Model file for the job. Use its own axes, mm. Coordinates: 2 decimals unless noted, no trailing zeros. Loops run counter-clockwise (first coordinate to the right, second up) from the corner with the lowest first, then second, coordinate; pieces in that order, holes last.
from build123d import *

# Parameters (mm, degrees)
SKETCH1_R           = 2.5
BOSS_EXTRUDE1_DEPTH = 9


with BuildPart() as part:
    # Sketch1 → Boss-Extrude1 (new body)
    # profile 1 of 2: a face of its own
    with BuildSketch(Plane(origin=(0, 0, 0), x_dir=(1, 0, 0), z_dir=(0, 1, 0))):
        Polygon((42.5, 102.604076401), (-42.5, 102.604076401), (-102.604076401, 42.5), (-102.604076401, -42.5), (-42.5, -102.604076401), (42.5, -102.604076401), (102.604076401, -42.5), (102.604076401, 42.5), align=None)
        with Locations(Location((-39.448264129, -95.209016687, 0), (0, 0, 270))):
            Circle(SKETCH1_R, mode=Mode.SUBTRACT)
        with BuildLine():
            Line((-59.824116139, -64.773863607), (-64.066756826, -69.016504294))
            ThreePointArc((-64.066756826, -69.016504294), (-69.016504294, -69.016504294), (-69.016504294, -64.066756826))
            Line((-69.016504294, -64.066756826), (-64.773863607, -59.824116139))
            ThreePointArc((-64.773863607, -59.824116139), (-60.95959786, -59.065411509), (-58.798989873, -62.298989873))
            ThreePointArc((-58.798989873, -62.298989873), (-59.065411509, -63.638381887), (-59.824116139, -64.773863607))
        make_face(mode=Mode.SUBTRACT)
        with Locations(Location((39.428806258, -95.217076401, 0), (0, 0, 270))):
            Circle(SKETCH1_R, mode=Mode.SUBTRACT)
        with Locations(Location((-95.217076401, -39.428806258, 0), (0, 0, 270))):
            Circle(SKETCH1_R, mode=Mode.SUBTRACT)
        with BuildLine():
            Line((64.773863607, -59.824116139), (69.016504294, -64.066756826))
            ThreePointArc((69.016504294, -64.066756826), (69.775208924, -65.202238547), (70.04163056, -66.54163056))
            ThreePointArc((70.04163056, -66.54163056), (67.881022574, -69.775208924), (64.066756826, -69.016504294))
            Line((64.066756826, -69.016504294), (59.824116139, -64.773863607))
            ThreePointArc((59.824116139, -64.773863607), (59.824116139, -59.824116139), (64.773863607, -59.824116139))
        make_face(mode=Mode.SUBTRACT)
        with Locations(Location((95.209016687, -39.448264129, 0), (0, 0, 270))):
            Circle(SKETCH1_R, mode=Mode.SUBTRACT)
        with Locations(Location((-95.209016687, 39.448264129, 0), (0, 0, 270))):
            Circle(SKETCH1_R, mode=Mode.SUBTRACT)
        with BuildLine():
            Line((-64.773863607, 59.824116139), (-69.016504294, 64.066756826))
            ThreePointArc((-69.016504294, 64.066756826), (-69.016504294, 69.016504294), (-64.066756826, 69.016504294))
            Line((-64.066756826, 69.016504294), (-59.824116139, 64.773863607))
            ThreePointArc((-59.824116139, 64.773863607), (-59.065411509, 63.638381887), (-58.798989873, 62.298989873))
            ThreePointArc((-58.798989873, 62.298989873), (-60.95959786, 59.065411509), (-64.773863607, 59.824116139))
        make_face(mode=Mode.SUBTRACT)
        with Locations(Location((-39.428806258, 95.217076401, 0), (0, 0, 270))):
            Circle(SKETCH1_R, mode=Mode.SUBTRACT)
        with Locations(Location((39.448264129, 95.209016687, 0), (0, 0, 270))):
            Circle(SKETCH1_R, mode=Mode.SUBTRACT)
        with Locations(Location((95.217076401, 39.428806258, 0), (0, 0, 270))):
            Circle(SKETCH1_R, mode=Mode.SUBTRACT)
        with BuildLine():
            Line((59.824116139, 64.773863607), (64.066756826, 69.016504294))
            ThreePointArc((64.066756826, 69.016504294), (67.881022574, 69.775208924), (70.04163056, 66.54163056))
            ThreePointArc((70.04163056, 66.54163056), (69.775208924, 65.202238547), (69.016504294, 64.066756826))
            Line((69.016504294, 64.066756826), (64.773863607, 59.824116139))
            ThreePointArc((64.773863607, 59.824116139), (59.824116139, 59.824116139), (59.824116139, 64.773863607))
        make_face(mode=Mode.SUBTRACT)
    # profile 2 of 2: a face of its own
    with BuildSketch(Plane(origin=(0, 0, 0), x_dir=(1, 0, 0), z_dir=(0, 1, 0))):
        Polygon((102.604076401, -42.5), (185.604076401, -42.5), (210.604076401, -17.5), (210.604076401, 17.5), (185.604076401, 42.5), (102.604076401, 42.5), align=None)
    extrude(amount=BOSS_EXTRUDE1_DEPTH)


solid = part.part
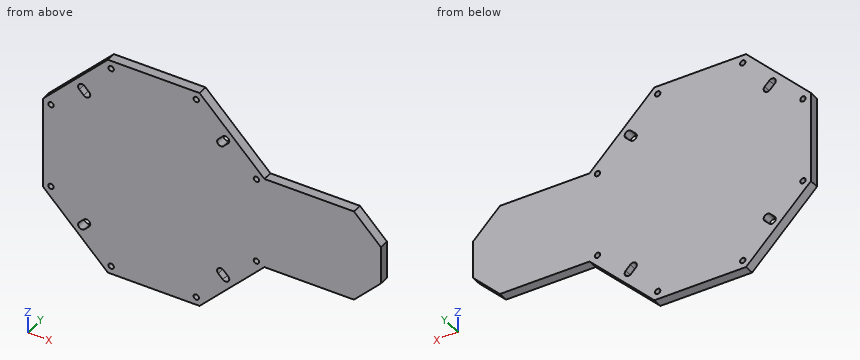
Q1. Slice it at B-B (y = 3.25). Count the separate pieces of the cut face and the enclosed holes in it, and give its area (3 significant figures).
Answers:
separate pieces: 1
enclosed holes: 12
area: 43,000 mm2
Q2. Flat gauge pins, fed straight in: P1, Ø5, axis at y = 6.5, z = 63, coming from the +X side; P2, Ø1, axis at y = 3, z = -68, coming from the +X side; P3, Ø6, axis at x = 39.43, z = 95.22, coming from the +Y side; P4, Ø4, axis at y = 6.5, z = -54, coming from the +X side. Where does each tip first touch, or does it go through?
Answers:
P1: stops at x = 84.6
P2: stops at x = 77.6
P3: stops at y = 9
P4: stops at x = 93.1
Q3. Drill centre lines: line 1 (X direction, y = 8.5, z = -68); line 2 (Z direction, x = 67, y = 5); line 3 (Z direction, x = 63, y = 6). Where is each one in solid material? Low to high.
Answers:
line 1: x = -77.1 to -69.72, -63.05 to 63.05, 69.72 to 77.1
line 2: z = -78.1 to -70.01, -62.05 to 62.05, 70.01 to 78.1
line 3: z = -82.1 to -67.95, -58.87 to 58.87, 67.95 to 82.1
Q4. Slice it at C-C (z = 81.5). List the corners of the cut face in (x, y).
Answers:
outline: (-63.6, 0) - (63.6, 0) - (63.6, 9) - (-63.6, 9) - close
Q5. Slice it at A-A (x = 160). List the corners of the cut face in (y, z).
Answers:
outline: (0, -42.5) - (9, -42.5) - (9, 42.5) - (0, 42.5) - close
